Build history of the part. All positions in model axes, mm. Face numbers are marked on the shaded views. A direction names the side the tool comes from. Coordinates: 2 decimals unless noted, no trailing zeros. Write each loop counter-clockwise with the first axis right and the second up, starting at its lowest first coordinate (ties: lowest second). Pieces come first, ordered by that corner, then holes.
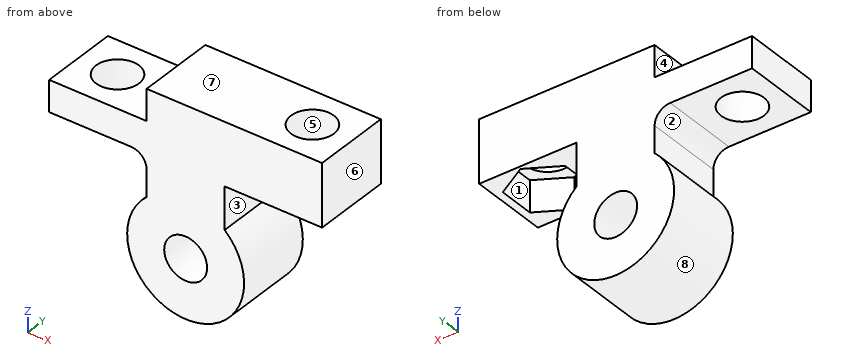
Autodesk Inventor part; units mm, degrees
ref_plane "YZ Plane" through (0, 0, 0) normal (1, 0, 0) x (0, 1, 0)
ref_plane "XZ Plane" through (0, 0, 0) normal (0, 1, 0) x (-1, 0, 0)
ref_plane "XY Plane" through (0, 0, 0) normal (0, 0, 1) x (1, 0, 0)
sketch "Sketch4" plane through (0, 0, 0) normal (0, 1, 0) x (-1, 0, 0)
  circle A0 centre (0, 0) radius 7.5
  circle A1 centre (0, 0) radius 2.75
  dimension "d19" = 15
  dimension "d20" = 5.5
extrude "Extrusion4" add sketch "Sketch4" along normal blind 10
ref_plane "Work Plane1" through (0, 10, 0) normal (0, -1, 0) x (1, 0, 0)
sketch "Sketch7" plane through (0, 10, 0) normal (0, -1, 0) x (1, 0, 0)
  line L0 (0, 0) -> (0, 15)
  line L1 (17.5, 19) -> (-17.5, 19)
  line L2 (-17.5, 19) -> (-17.5, 11)
  line L3 (-17.5, 11) -> (17.5, 11)
  line L4 (17.5, 11) -> (17.5, 19)
  line L5 (17.5, 19) -> (-17.5, 11) construction
  line L6 (-17.5, 19) -> (17.5, 11) construction
  line L7 (5, 24.41) -> (-5, 24.41)
  line L8 (-5, 24.41) -> (-5, 5.59)
  line L9 (-5, 5.59) -> (5, 5.59)
  line L10 (5, 5.59) -> (5, 24.41)
  line L11 (5, 24.41) -> (-5, 5.59) construction
  line L12 (-5, 24.41) -> (5, 5.59) construction
  point P0 (-5, 11)
  point P1 (5, 11)
  dimension "d35" = 15
  dimension "d36" = 35
  dimension "d37" = 8
  dimension "d38" = 10
  dimension "d39" = 18.82
extrude "Extrusion6" add sketch "Sketch7" along normal up to surface (10 mm away) contours L9 L8 L3 L0 | L0 L3 L10 L9 | L3 L8 L1 L10 | L3 L2 L1 L8 | L10 L1 L4 L3
sketch "Sketch8" plane through (-5, 10, 11) normal (0, 0, -1) x (-1, 0, 0)
  point P0 (-5, -10)
sketch "Sketch10" plane through (17.5, 10, 11) normal (0, 0, -1) x (-1, 0, 0)
  circle A0 centre (5, -5) radius 2.75
  circle A1 centre (30, -5) radius 2.75
  line L0 (35, -10) -> (22.5, -10)
  line L1 (35, 0) -> (35, -10)
  line L2 (0, 0) -> (0, -10)
  line L3 (12.5, -10) -> (0, -10)
  point P0 (17.5, -10)
  dimension "d50" = 5.5
  dimension "d51" = 5.5
  dimension "d52" = 5
  dimension "d53" = 5
  dimension "d54" = 5
  dimension "d55" = 5
extrude "Extrusion8" cut sketch "Sketch10" against normal through all
sketch "Sketch11" plane through (17.5, 10, 11) normal (0, 0, -1) x (-1, 0, 0)
  circle A0 centre (5, -5) radius 2.75
  line L0 (5, -9.6188) -> (1, -7.3094)
  line L1 (1, -7.3094) -> (1, -2.6906)
  line L2 (1, -2.6906) -> (5, -0.3812)
  line L3 (5, -0.3812) -> (9, -2.6906)
  line L4 (9, -2.6906) -> (9, -7.3094)
  line L5 (9, -7.3094) -> (5, -9.6188)
  line L6 (0, 0) -> (0, -10)
  line L7 (12.5, 0) -> (12.5, -10)
  line L8 (0, 0) -> (12.5, 0)
  line L9 (12.5, 0) -> (12.5, -10)
  line L10 (12.5, -10) -> (0, -10)
  line L11 (0, -10) -> (0, 0)
  point P0 (17.5, -10)
  point P1 (12.4201, 0)
  dimension "d58" = 8
fillet "Fillet3" radius 2 1 edges at (-5, 5, 11)
extrude "Extrusion10" cut sketch "Sketch11" against normal blind 4 contours L0 L1 L2 L3 L4 L5
sketch "Sketch12" plane through (17.5, 0, 19) normal (0, 0, 1) x (1, 0, 0)
  line L0 (-22.5, 0) -> (-22.5, 10)
  line L1 (-35, 10) -> (-35, 0)
  line L2 (-22.5, 0) -> (-35, 0)
  line L3 (-35, 0) -> (-35, 10)
  line L4 (-35, 10) -> (-22.5, 10)
  line L5 (-22.5, 10) -> (-22.5, 0)
  point P0 (-17.5, 0)
extrude "Extrusion11" cut sketch "Sketch12" against normal blind 4
properties part number "4mm_Roller_Spacer_R" material "PET Plastic"
1. Saw through at A-A on y = 5. List the corners of the cut face in (x, z), plus the area to 3 significant figures.
Computed values:
outline: (-17.5, 11) - (-15.25, 11) - (-15.25, 15) - (-17.5, 15) - close; (-9.75, 11) - (-7, 11) arc R2 cw to (-5, 9) - (-5, 5.59) arc R7.5 ccw (long way) to (5, 5.59) - (5, 11) - (8.5, 11) - (8.5, 15) - (9.75, 15) - (9.75, 19) - (-5, 19) - (-5, 15) - (-9.75, 15) - close; (15.25, 15) - (16.5, 15) - (16.5, 11) - (17.5, 11) - (17.5, 19) - (15.25, 19) - close; hole circle Ø5.5 at (0, 0)
area: 349 mm2
2. Mould opens along Z. For the marked faces 6, 7 and 8 say: +Z half, -Z half, draft (parallel to the pull), parting line (faces both ways), or undercut.
Computed values:
face 6: draft
face 7: +Z half
face 8: undercut
3. Saw through at D-D on z = 12. List the corners of the cut face in (x, y), plus the area to 3 significant figures.
Computed values:
outline: (-17.5, 0) - (17.5, 0) - (17.5, 10) - (-17.5, 10) - close; hole circle Ø5.5 at (-12.5, 5); hole (8.5, 2.69) - (12.5, 0.38) - (16.5, 2.69) - (16.5, 7.31) - (12.5, 9.62) - (8.5, 7.31) - close
area: 271 mm2
4. Saw through at C-C on x = -12.5. List the corners of the cut face in (y, z).
Computed values:
outline: (0, 11) - (2.25, 11) - (2.25, 15) - (0, 15) - close; (7.75, 11) - (10, 11) - (10, 15) - (7.75, 15) - close
5. Saw through at B-B on z = 0. List the corners of the cut face in (x, y).
Computed values:
outline: (-7.5, 0) - (-2.75, 0) - (-2.75, 10) - (-7.5, 10) - close; (2.75, 0) - (7.5, 0) - (7.5, 10) - (2.75, 10) - close
6. Flat gauge pins, fed straight in: pin 1 (6 mm diameter, centred on y = 6.5, z = 7.5, fed in from +X); pin 2 (3 mm diameter, centred on x = 13, y = 7, fed in from -Z); pin 3 (6 mm diameter, centred on y = 4, z = 7, fed in from -X). Where does each tip first touch, or does it go through?
Computed values:
pin 1: stops at x = 6
pin 2: stops at z = 15
pin 3: stops at x = -6.34
7. Probe line 1 along Y through (x, z) = (-12.5, 13.3); line 2 along Z through (x, y) = (0, 2); line 3 along Z through (x, y) = (12, 1.75). List the from-to ranges inside material, lowest first.
Computed values:
line 1: y = 0 to 2.25, 7.75 to 10
line 2: z = -7.5 to -2.75, 2.75 to 19
line 3: z = 15 to 19
8. 3-axis set-ups, long thin cutter, end or side, ignore diameter. For the marked faces 1, 2, 3, 4 and 5: which of +Z, -Z, +X, -X, +Y, -Y reach the whole face in a straight line?
Computed values:
face 1: -Z
face 2: -X, +Y, -Y
face 3: +X, +Y, -Y
face 4: +Z, -X, +Y, -Y
face 5: +Z, -Z
